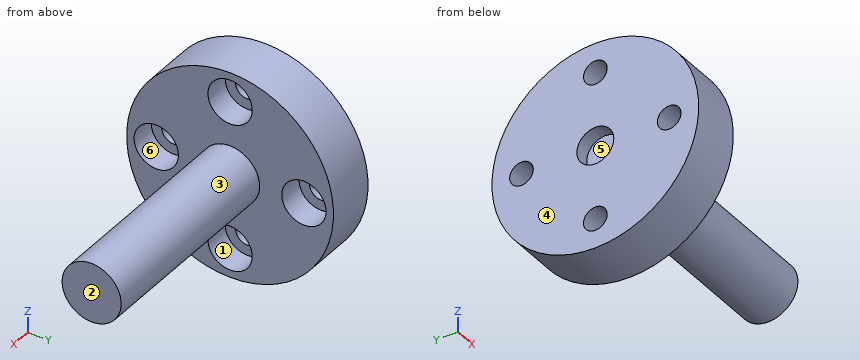
from build123d import *

# Parameters (mm, degrees)
CBORE_FOR_M3_SBHCS1_D           = 3.2
CBORE_FOR_M3_SBHCS1_CBORE_D     = 6
CBORE_FOR_M3_SBHCS1_CBORE_DEPTH = 3.5
CIRPATTERN1_COUNT               = 4
SKETCH5_R                       = 2.5
CUT_EXTRUDE1_DEPTH              = 2


with BuildPart() as part:
    # Sketch2 → Revolve2 (revolve)
    with BuildSketch(Plane.XY, mode=Mode.PRIVATE) as revolve2_sk:
        Polygon((0, 14), (0, 0), (35, 0), (35, 4), (7, 4), (7, 14), align=None)
    revolve(revolve2_sk.sketch.rotate(Axis((0, 0, 0), (1, 0, 0)), 90), axis=Axis((0, 0, 0), (1, 0, 0)))

    # CBORE for M3 SBHCS1 (through all)
    with Locations(Plane(origin=(7, 0, 0), x_dir=(0, 0, -1), z_dir=(1, 0, 0))):
        with Locations((10, 0)):
            cbore_for_m3_sbhcs1 = CounterBoreHole(CBORE_FOR_M3_SBHCS1_D / 2, CBORE_FOR_M3_SBHCS1_CBORE_D / 2, CBORE_FOR_M3_SBHCS1_CBORE_DEPTH)

    # CirPattern1: CBORE for M3 SBHCS1 ×4 about axis
    cirpattern1_axis = Axis((0, 0, 0), (1, 0, 0))
    for i in range(1, CIRPATTERN1_COUNT):
        add(cbore_for_m3_sbhcs1.rotate(cirpattern1_axis, i * 360 / CIRPATTERN1_COUNT), mode=Mode.SUBTRACT)

    # Sketch5 → Cut-Extrude1 (cut)
    with BuildSketch(Plane.ZY):
        Circle(SKETCH5_R)
    extrude(amount=-CUT_EXTRUDE1_DEPTH, mode=Mode.SUBTRACT)


solid = part.part
The listing builds one solid part. Answer for the finished solid, in the listing's coordinates (mm). Face numbers are marked on the shaded views. A direction names the side the tool comes from. Round coordinates to 2 decimals unless told otherwise and drop trailing zeros. Write each loop counter-clockwise with the first axis right and the second up, starting at its lowest first coordinate (ties: lowest second). Pieces come first, ordered by that corner, then holes. Notation, with made-up numbers: M 66,0 L 89,0 A8 ccw 89,5 Z; hole C -31,11 d6. An arc over 180 degrees is marked long. Write each question's results on one line, items separated by ' | '. Start each with the question number.
Item 1: Given pin 1 Ø10 at (x, y) = (18.5, 0) entering from +Z; pin 2 Ø1.5 at (y, z) = (-1, 0) entering from -X; pin 3 Ø9.5 at (y, z) = (-10, 0) entering from +X; pin 4 Ø1.9 at (y, z) = (-10, 0) entering from -X, each flat-ended and moving along its own axis, determine where each tip first touches the part or whether it passes through.
Item 2: Find section A-A on z = 10. Write down the section's boundary in (x, y), and give its area (3 significant figures).
Item 3: Straight lines are drawn through the part: probe 1 along X at (y, z) = (12, 2.5); probe 2 along X at (y, z) = (1.5, 0.25); probe 3 along Z at (x, y) = (1.55, -10). For each, find the intervals that lie inside material, in ascending order.
Item 4: Which of the six approach directions +Z, -Z, +X, -X, +Y, -Y give full straight-line access (tool end or side, diameter ignored) to the marked faces 4, 5 and 6?
Item 5: Find section C-C on x = 15. Write down the section's boundary in (y, z), and give its area (3 significant figures).
Item 6: The mould has two halves that part along Y. Classify the marked faces 1, 2 and 3: +Y half, -Y half, draft (parallel to the pull), parting line (faces both ways), or undercut.
Item 7: Find section D-D on z = 5. Write down the section's boundary in (x, y).
Answer block:
1) pin 1: stops at z = 4 | pin 2: stops at x = 2 | pin 3: stops at x = 7 | pin 4: passes through
2) outline: M 0,-9.8 L 7,-9.8 L 7,-3 L 3.5,-3 L 3.5,-1.6 L 0,-1.6 Z; M 0,1.6 L 3.5,1.6 L 3.5,3 L 7,3 L 7,9.8 L 0,9.8 Z | area: 105 mm²
3) probe 1: x = 0 to 7 | probe 2: x = 2 to 35 | probe 3: z = -9.8 to -1.6, 1.6 to 9.8
4) face 4: +Z, -Z, -X, +Y, -Y | face 5: -X | face 6: +X
5) outline: C 0,0 d8 | area: 50.3 mm²
6) face 1: undercut | face 2: draft | face 3: parting line
7) outline: M 0,-13.08 L 7,-13.08 L 7,13.08 L 0,13.08 Z
